from build123d import *

# Parameters (mm, degrees)
F0_R     = 25
F1_DEPTH = 5
F2_R     = 6.25
F3_DEPTH = 49.5
F4_R     = 20
F5_DEPTH = 5
F6_R     = 2.75
F7_DEPTH = 5


with BuildPart() as f1:
    # F0 (on Top) → F1 (new body)
    with BuildSketch(Plane.XY):
        Circle(F0_R)
    extrude(amount=F1_DEPTH)

    # F2 (on face) → F3 (join)
    with BuildSketch(Plane.XY.offset(5)):
        Circle(F2_R)
    extrude(amount=F3_DEPTH)

    # F4 (on face) → F5 (join)
    with BuildSketch(Plane.XY.offset(54.5)):
        Circle(F4_R)
    extrude(amount=F5_DEPTH)

    # F6 (on face) → F7 (cut)
    with BuildSketch(Plane.XY.offset(59.5)):
        with Locations((0, 15)):
            Circle(F6_R)
        with Locations((15, 0)):
            Circle(F6_R)
        with Locations((0, -15)):
            Circle(F6_R)
        with Locations((-15, 0)):
            Circle(F6_R)
    extrude(amount=-F7_DEPTH, mode=Mode.SUBTRACT)


solid = f1.part
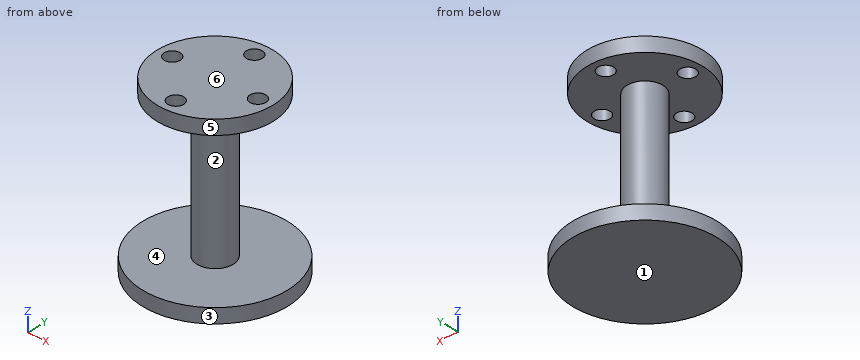
CAD build for the part. Positions are in the model's coordinates, mm. Face numbers are marked on the shaded views. A direction names the side the tool comes from. Give positions to 0.01 mm unless a question says otherwise; leave off trailing zeros. Order: outer loops, then holes, each group sorted by start corner. A loop starts at its lowest first (then second) coordinate and runs counter-clockwise, first axis right, second up. Notation, with made-up numbers: (56.25, -19) - (65.25, -19) arc R33 cw to (65.25, 16) - close; hole circle Ø5 at (-15.75, 57). An arc over 180 degrees is marked (long way). Answer in a Markdown table with one row per item.
1. Probe probe 1 along Y at (x, z) = (0, 56.8); probe 2 along Z at (x, y) = (-12, -12.5); probe 3 along Y at (x, z) = (15, 56.75). List the from-to ranges inside material, lowest first. Write a range as [from, to].
Data:
| item | result |
|---|---|
| probe 1 | y = [-20, -17.75], [-12.25, 12.25], [17.75, 20] |
| probe 2 | z = [0, 5], [54.5, 59.5] |
| probe 3 | y = [-13.23, -2.75], [2.75, 13.23] |
2. Saw through at A-A, the plane y = 0. Give the cut face in (x, z).
Data:
| item | result |
|---|---|
| outline | (-25, 0) - (25, 0) - (25, 5) - (6.25, 5) - (6.25, 54.5) - (12.25, 54.5) - (12.25, 59.5) - (-12.25, 59.5) - (-12.25, 54.5) - (-6.25, 54.5) - (-6.25, 5) - (-25, 5) - close; (-20, 54.5) - (-17.75, 54.5) - (-17.75, 59.5) - (-20, 59.5) - close; (17.75, 54.5) - (20, 54.5) - (20, 59.5) - (17.75, 59.5) - close |
3. Flat gauge pins, fed straight in: pin 1 (12 mm diameter, centred on y = -17.5, z = 30.5, fed in from +X); pin 2 (10 mm diameter, centred on y = -5.5, z = 39.5, fed in from -X); pin 3 (5 mm diameter, centred on x = 0, y = 15, fed in from +Z). Where does each tip first touch, or does it go through?
Data:
| item | result |
|---|---|
| pin 1 | passes through |
| pin 2 | stops at x = -6.23 |
| pin 3 | stops at z = 5 |
4. Pull direction Z, two halves, no side cores. Call the marked faces 1, 2 and 3: pulls with the +Z half, pulls with the -Z half, needs draft (parallel to the pull), parting line crosses it, or undercut.
Data:
| item | result |
|---|---|
| face 1 | pulls with the -Z half |
| face 2 | undercut |
| face 3 | needs draft |
5. Saw through at B-B, the plane x = 16.5. Give the cut face in (y, z).
Data:
| item | result |
|---|---|
| outline | (-18.78, 0) - (18.78, 0) - (18.78, 5) - (-18.78, 5) - close; (-11.3, 54.5) - (-2.3, 54.5) - (-2.3, 59.5) - (-11.3, 59.5) - close; (2.3, 54.5) - (11.3, 54.5) - (11.3, 59.5) - (2.3, 59.5) - close |
6. Tool access for the marked faces 4, 5 and 6: list every direction of +Z, -Z, +X, -X, +Y, -Y with a clear straight run to the whole face (end or side of a thin tool).
Data:
| item | result |
|---|---|
| face 4 | none |
| face 5 | +Z |
| face 6 | +Z, +X, -X, +Y, -Y |
7. Saw through at C-C, the plane y = 10. Give the cut face in (x, z).
Data:
| item | result |
|---|---|
| outline | (-22.91, 0) - (22.91, 0) - (22.91, 5) - (-22.91, 5) - close; (-17.32, 54.5) - (17.32, 54.5) - (17.32, 59.5) - (-17.32, 59.5) - close |
